Geometry check sheet. Reference: the model listing, model coordinates, mm. Face numbers are marked on the shaded views. A direction names the side the tool comes from. Give positions to 0.01 mm unless a question says otherwise; leave off trailing zeros. Order: outer loops, then holes, each group sorted by start corner. A loop starts at its lowest first (then second) coordinate and runs counter-clockwise, first axis right, second up.
Autodesk Inventor part; units mm, degrees
ref_plane "Work Plane1" through (-29, 0, 0) normal (1, 0, 0) x (0, 0, -1)
ref_plane "YZ Plane" through (0, 0, 0) normal (1, 0, 0) x (0, 1, 0)
ref_plane "XZ Plane" through (0, 0, 0) normal (0, 1, 0) x (-1, 0, 0)
sketch "Sketch1" plane through (0, 0, 0) normal (1, 0, 0) x (0, 1, 0)
  circle A0 centre (0, 0) radius 19.25
  circle A1 centre (0, 0) radius 17.25
  circle A2 centre (0, 0) radius 22.25
  dimension "d0" = 38.5
  dimension "d1" = 34.5
  dimension "d6" = 44.5
extrude "Extrusion1" add sketch "Sketch1" along normal blind 5 contours A0 | A1 | A2
extrude "Extrusion2" add sketch "Sketch1" against normal blind 71 contours A1
extrude "Extrusion3" add sketch "Sketch1" against normal blind 34 contours A2
sketch "Sketch2" plane through (5, 0, 0) normal (1, 0, 0) x (0, 0, -1)
  line L0 (0, -7.5) -> (-6.4952, -3.75)
  line L1 (-6.4952, -3.75) -> (-6.4952, 3.75)
  line L2 (-6.4952, 3.75) -> (0, 7.5)
  line L3 (0, 7.5) -> (6.4952, 3.75)
  line L4 (6.4952, 3.75) -> (6.4952, -3.75)
  line L5 (6.4952, -3.75) -> (0, -7.5)
extrude "Extrusion4" cut sketch "Sketch2" against normal through all
sketch "Sketch3" plane through (-34, 0, 0) normal (-1, 0, 0) x (0, 0, 1)
  circle A0 centre (0, 0) radius 42.5
  circle A1 centre (0, 0) radius 22.25
  dimension "d12" = 85
extrude "Extrusion5" add sketch "Sketch3" against normal blind 5
sketch "Sketch4" plane through (5, 0, 0) normal (1, 0, 0) x (0, 0, -1)
  line L0 (0, -7.5) -> (-6.4952, -3.75)
  line L1 (-6.4952, -3.75) -> (-6.4952, 3.75)
  line L2 (-6.4952, 3.75) -> (0, 7.5)
  line L3 (0, 7.5) -> (6.4952, 3.75)
  line L4 (6.4952, 3.75) -> (6.4952, -3.75)
  line L5 (6.4952, -3.75) -> (0, -7.5)
  circle A0 centre (0, 0) radius 4.05
  dimension "d15" = 8.1
extrude "Extrusion6" add sketch "Sketch4" against normal blind 4
ref_plane "Work Plane1" through (-29, 0, 0) normal (1, 0, 0) x (0, 0, -1)
sketch "Sketch5" plane through (-29, 0, 0) normal (1, 0, 0) x (0, 0, -1)
  line L0 (0, 0) -> (34.5, 0)
  circle A0 centre (34.5, 0) radius 4.05
  circle A1 centre (0, 34.5) radius 4.05
  circle A2 centre (-34.5, 0) radius 4.05
  circle A3 centre (0, -34.5) radius 4.05
  dimension "d19" = 34.5
  dimension "d20" = 8.1
  dimension "d23" = 360
extrude "Extrusion7" cut sketch "Sketch5" against normal up to surface (5 mm away)
sketch "Sketch6" plane through (5, 0, 0) normal (1, 0, 0) x (0, 0, -1)
  circle A0 centre (0, 0) radius 22.25
  circle A1 centre (0, 0) radius 23.25
  dimension "d27" = 46.5
extrude "Extrusion8" add sketch "Sketch6" against normal up to surface (34 mm away)
sketch "Sketch7" plane through (5, 0, 0) normal (1, 0, 0) x (0, 0, -1)
  circle A0 centre (0, 0) radius 23.25
  circle A1 centre (0, -34.5) radius 4.05
  circle A2 centre (0, 34.5) radius 4.05
  circle A3 centre (34.5, 0) radius 4.05
  circle A4 centre (-34.5, 0) radius 4.05
  circle A5 centre (0, 0) radius 42.5
extrude "Extrusion9" add sketch "Sketch7" against normal blind 5
sketch "Sketch8" plane through (-34, 0, 0) normal (-1, 0, 0) x (0, 0, 1)
  circle A0 centre (0, -34.5) radius 4.05
  circle A1 centre (0, 34.5) radius 4.05
  circle A2 centre (-34.5, 0) radius 4.05
  circle A3 centre (34.5, 0) radius 4.05
  circle A4 centre (0, 0) radius 42.5
  circle A5 centre (0, 0) radius 19.25
extrude "Extrusion10" cut sketch "Sketch8" against normal up to surface (5 mm away)
sketch "Sketch9" plane through (5, 0, 0) normal (1, 0, 0) x (0, 0, -1)
  circle A0 centre (0, -34.5) radius 4.05
  circle A1 centre (0, 34.5) radius 4.05
  circle A2 centre (34.5, 0) radius 4.05
  circle A3 centre (-34.5, 0) radius 4.05
  circle A4 centre (0, 0) radius 42.5
  circle A5 centre (0, 0) radius 4.05
extrude "Extrusion11" add sketch "Sketch9" along normal blind 1
sketch "Sketch10" plane through (0, 0, 0) normal (-1, 0, 0) x (0, 0, 1)
  circle A0 centre (0, 0) radius 42.5
  circle A1 centre (34.5, 0) radius 4.05
  circle A2 centre (-34.5, 0) radius 4.05
  circle A3 centre (0, 34.5) radius 4.05
  circle A4 centre (0, -34.5) radius 4.05
  circle A5 centre (0, 0) radius 23.25
extrude "Extrusion12" add sketch "Sketch10" along normal blind 2.5
sketch "Sketch11" plane through (6, 0, 0) normal (1, 0, 0) x (0, 0, -1)
  circle A0 centre (0, 34.5) radius 4.05
  line L0 (-4.05, 34.5) -> (-4.05, 42.3066)
  line L1 (4.05, 34.5) -> (4.05, 42.3066)
  circle A1 centre (0, 0) radius 42.5
  arc A2 (4.05, 34.5) -> (-4.05, 34.5) centre (0, 34.5) ccw
  circle A3 centre (0, 0) radius 4.05
  arc A4 (4.05, 42.3066) -> (-4.05, 42.3066) centre (0, 0) ccw
  line L2 (-34.5, -4.05) -> (-42.3066, -4.05)
  line L3 (-34.5, 4.05) -> (-42.3066, 4.05)
  arc A5 (-34.5, 4.05) -> (-34.5, -4.05) centre (-34.5, 0) ccw
  arc A6 (-42.3066, 4.05) -> (-42.3066, -4.05) centre (0, 0) ccw
  line L4 (4.05, -34.5) -> (4.05, -42.3066)
  line L5 (-4.05, -34.5) -> (-4.05, -42.3066)
  arc A7 (-4.05, -34.5) -> (4.05, -34.5) centre (0, -34.5) ccw
  arc A8 (-4.05, -42.3066) -> (4.05, -42.3066) centre (0, 0) ccw
  line L6 (34.5, 4.05) -> (42.3066, 4.05)
  line L7 (34.5, -4.05) -> (42.3066, -4.05)
  arc A9 (34.5, -4.05) -> (34.5, 4.05) centre (34.5, 0) ccw
  arc A10 (42.3066, -4.05) -> (42.3066, 4.05) centre (0, 0) ccw
  dimension "d40" = 360
extrude "Extrusion13" cut sketch "Sketch11" against normal up to surface (8.5 mm away) contours A0 L0 A1 L1 | A1 L7 A9 L6 | L3 A5 L2 A1 | L5 A7 L4 A1
sketch "Sketch12" plane through (1, 0, 0) normal (-1, 0, 0) x (0, 0, 1)
  point P0 (0, 0)
properties part number "wheel_adapter_inner"
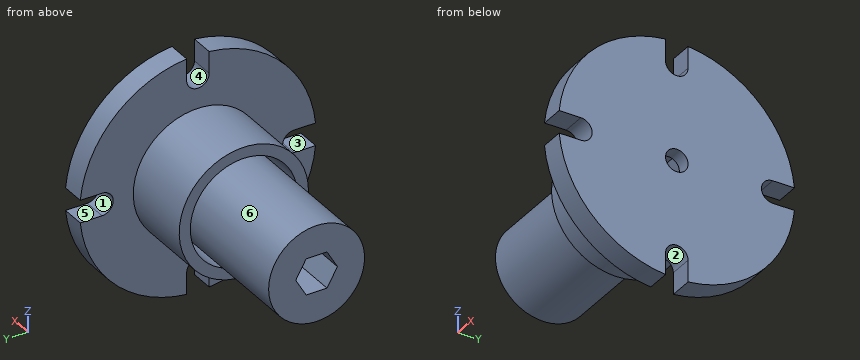
Item 1: Sectioned sample at B-B (y = 0). Enter the section's corners in (x, z).
Reported:
outline: (-71, -17.25) - (0, -17.25) - (0, -19.25) - (-29, -19.25) - (-29, -23.25) - (-2.5, -23.25) - (-2.5, -30.45) - (6, -30.45) - (6, -4.05) - (1, -4.05) - (1, -6.5) - (-71, -6.5) - close; (-71, 6.5) - (1, 6.5) - (1, 4.05) - (6, 4.05) - (6, 30.45) - (-2.5, 30.45) - (-2.5, 23.25) - (-29, 23.25) - (-29, 19.25) - (0, 19.25) - (0, 17.25) - (-71, 17.25) - close
Item 2: Gauge pin test, flat ends, axial feed: pin 1 (8.5 mm diameter, centred on x = 3, z = -39.5, fed in from +Y); pin 2 (8 mm diameter, centred on x = -58, y = 14, fed in from +Z); pin 3 (8.5 mm diameter, centred on x = 1.5, y = -38.5, fed in from -Z); pin 4 (14.5 mm diameter, centred on y = 1.5, z = -1.5, fed in from -X). Record the tip position at first contact, or that the pin passes through.
Reported:
pin 1: stops at y = 23.74
pin 2: stops at z = 14.06
pin 3: stops at z = -25.16
pin 4: stops at x = -71
Item 3: Draft check along Y on the marked faces 1, 2 and 3. Enter one of: released by +Y, released by -Y, zero draft, split by the parting line, or undercut.
Reported:
face 1: released by +Y
face 2: undercut
face 3: zero draft
Item 4: Sectioned sample at A-A (x = -63). Enter the section's corners in (y, z), and give its area (3 significant figures).
Reported:
outline: circle Ø34.5 at (0, 0); hole (-7.5, 0) - (-3.75, -6.5) - (3.75, -6.5) - (7.5, 0) - (3.75, 6.5) - (-3.75, 6.5) - close
area: 789 mm2
Item 5: Scan lines: L1, parallel to Y at x = 3.75, z = 0; L2, parallel to Z at x = -1, y = -12; L3, parallel to X at y = -37, z = 8. Record each from-to range of solid material in increasing order.
Reported:
L1: y = -30.45 to -4.05, 4.05 to 30.45
L2: z = -40.77 to -15.05, -12.39 to 12.39, 15.05 to 40.77
L3: x = -2.5 to 6
Item 6: Sectioned sample at D-D (y = 32). Enter the section's corners in (x, z), and give its area (3 significant figures).
Reported:
outline: (-2.5, -27.97) - (6, -27.97) - (6, -3.19) - (-2.5, -3.19) - close; (-2.5, 3.19) - (6, 3.19) - (6, 27.97) - (-2.5, 27.97) - close
area: 421 mm2
Item 7: Set-up check for the marked faces 4, 5 and 6: record each of +Z, -Z, +X, -X, +Y, -Y from which the full face is reachable in a straight line by a thin tool's end or side.
Reported:
face 4: +Z, +X, -X
face 5: +X, -X, +Y
face 6: -X
Item 8: Sectioned sample at C-C (y = 21). Enter the section's corners in (x, z), and give its area (3 significant figures).
Reported:
outline: (-29, -9.98) - (-2.5, -9.98) - (-2.5, -36.95) - (6, -36.95) - (6, 36.95) - (-2.5, 36.95) - (-2.5, 9.98) - (-29, 9.98) - close
area: 1,160 mm2
